For this review, take the finished solid that the model builds, in its own axes (mm). Round coordinates to 2 decimals unless told otherwise and drop trailing zeros. Order: outer loops, then holes, each group sorted by start corner. A loop starts at its lowest first (then second) coordinate and runs counter-clockwise, first axis right, second up. Notation, with made-up numbers: M 4,-14 L 46,-14 A23 cw 46,24 Z; hole C 70.5,10.25 d8. An arc over 180 degrees is marked long. Answer as a JSON object with one key per item and string values.
from build123d import *

# Parameters (mm, degrees)
F0_W     = 25
F0_H     = 25
F1_DEPTH = 8
F2_W     = 1
F2_H     = 25
F3_DEPTH = 7
F4_W     = 1
F4_H     = 25
F5_DEPTH = 7.9
F6_R     = 3


with BuildPart() as f1:
    # F0 (on Front) → F1 (new body)
    with BuildSketch(Plane.XZ):
        with Locations((-0.469491, 0.276955)):
            Rectangle(F0_W, F0_H)
    extrude(amount=F1_DEPTH)

    # F2 (on face) → F3 (cut)
    with BuildSketch(Plane(origin=(-12.969491, 0, 0), x_dir=(0, -1, 0), z_dir=(-1, 0, 0))):
        with Locations((3.948362, 0.276955)):
            Rectangle(F2_W, F2_H)
    extrude(amount=-F3_DEPTH, mode=Mode.SUBTRACT)

    # F4 (on face) → F5 (cut)
    with BuildSketch(Plane.YZ.offset(12.030509)):
        with Locations((-4.006481, 0.276955)):
            Rectangle(F4_W, F4_H)
    extrude(amount=-F5_DEPTH, mode=Mode.SUBTRACT)

    # F6
    f6_edges = [f1.edges().sort_by_distance(p)[0] for p in [
        (-12.969491, -1.724181, 12.776955),
        (-12.969491, -6.224181, 12.776955),
        (12.030509, -6.25324, 12.776955),
        (12.030509, -1.75324, 12.776955),
        (12.030509, -6.25324, -12.223045),
        (12.030509, -1.75324, -12.223045),
        (-12.969491, -1.724181, -12.223045),
        (-12.969491, -6.224181, -12.223045),
    ]]
    fillet(f6_edges, radius=F6_R)


solid = f1.part
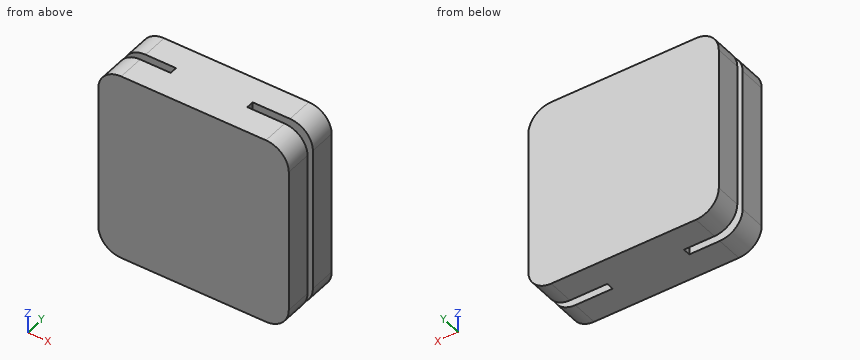
1) Add section B-B on z = -1.25. State the section outline as (x, y) points, and give its area (3 significant figures).
Geometry check:
{"outline": "M -12.97,-8 L 12.03,-8 L 12.03,-4.51 L 4.13,-4.51 L 4.13,-3.51 L 12.03,-3.51 L 12.03,0 L -12.97,0 L -12.97,-3.45 L -5.97,-3.45 L -5.97,-4.45 L -12.97,-4.45 Z", "area": "185 mm²"}
2) Insertion check: P1, Ø1, axis at x = -8, z = 7, coming from the +Y side; P2, Ø0.8, axis at y = -4, z = -3.5, coming from the +X side. Each pin has a flat end and moves straight along its axis. Give the tip position at first contact, or say it passes through.
Geometry check:
{"P1": "stops at y = 0", "P2": "stops at x = 4.13"}
3) For L1, parallel to Y at x = 4.5, z = 8; L2, parallel to Y at x = -6.25, z = 11.5; L3, parallel to X at y = -2.75, z = -10.25, list the stretches that pass through material, from the lowest coordinate up.
Geometry check:
{"L1": "y = -8 to -4.51, -3.51 to 0", "L2": "y = -8 to -4.45, -3.45 to 0", "L3": "x = -12.79 to 11.85"}
4) Add section C-C on x = 9.75. State the section outline as (y, z) points.
Geometry check:
{"outline": "M -8,-12.14 L -4.51,-12.14 L -4.51,12.69 L -8,12.69 Z; M -3.51,-12.14 L 0,-12.14 L 0,12.69 L -3.51,12.69 Z"}
5) Add section A-A on x = 5.75. State the section outline as (y, z) points, and give its area (3 significant figures).
Geometry check:
{"outline": "M -8,-12.22 L -4.51,-12.22 L -4.51,12.78 L -8,12.78 Z; M -3.51,-12.22 L 0,-12.22 L 0,12.78 L -3.51,12.78 Z", "area": "175 mm²"}
